Build history of the part. All positions in model axes, mm. A direction names the side the tool comes from. Give positions to 0.01 mm unless a question says otherwise; leave off trailing zeros. Order: outer loops, then holes, each group sorted by start corner. A loop starts at its lowest first (then second) coordinate and runs counter-clockwise, first axis right, second up. Notation, with made-up numbers: M -19.75,48.5 L 23.25,48.5 A18 ccw 23.25,72.5 Z; hole C -33,-37.5 d6. An arc over 180 degrees is marked long. Use CSV: the item, a comma, the result in double quotes. Start each with the question number.
Item 1: Band-saw the part on A-A on z = 0. Write the cut outline in (x, y).
Item 2: Band-saw the part on D-D on x = -32.5. Write the cut outline in (y, z), plus the area to 3 significant figures.
Item 3: Which spindle directions (+Z, -Z, +X, -X, +Y, -Y) get a long thin tool onto all of the face, cutting with end or side? Do faces 1 (the flat face through (19, 50.737, -19)), 2 (the cylindrical face through (0.1, 52.2, -28.5)), 3 (the conical face through (-12.376, 30.541, 3.897)). Say none if no direction does.
Item 4: Two-plate mould, pull along X, no slides. Class faces 4 (the cylindrical face through (-15.41, 56.78, -15.7)), 5 (the cylindrical face through (15.1, 56.8, 16)), 6 (the cylindrical face through (-28.5, 52.2, -0.1)): pulls with the +X half, pulls with the -X half, needs draft (parallel to the pull), parting line crosses it, or undercut.
Item 5: Wall check: line 1 along Z through (x, y) = (0, 54.25); line 2 along Z through (x, y) = (0, 12); line 3 along Y through (x, z) = (-28, -3). Give the ranges that are in metal, low to high.
Item 6: Band-saw the part on C-C on y = 9.5. Write the cut outline in (x, z), plus the area to 3 significant figures.
Item 7: Band-saw the part on B-B on x = 0. Write the cut outline in (y, z), plus the area to 3 significant figures.
Item 8: Pin check, flat tips, straight feed: P1, Ø1.4, axis at y = 52.5, z = -24, coming from the +X side; P2, Ø1.5, axis at y = 13, z = 9.5, coming from the -X side; P3, Ø12, axis at y = 14, z = 7, coming from the -X side. Stop position of each tip, or through.
from build123d import *

# Parameters (mm, degrees)
CUT_EXTRUDE1_START = -10
CUT_EXTRUDE1_DEPTH = 16
CIRPATTERN1_COUNT  = 2
CIRPATTERN1_ANGLE  = 90


with BuildPart() as part:
    # Sketch1 → Revolve1 (revolve)
    with BuildSketch(Plane.XY):
        with BuildLine():
            Line((-6.832916656, 22.5), (-6.832916656, 0))
            Line((-6.832916656, 0), (-8.332916656, 0))
            ThreePointArc((-8.332916656, 0), (-14, 11.25), (-8.332916656, 22.5))
            Line((-8.332916656, 22.5), (-24.635499254, 50.736901354))
            Line((-24.635499254, 50.736901354), (-45, 50.736901354))
            Line((-45, 50.736901354), (-45, 53.736901354))
            Line((-45, 53.736901354), (-22, 53.736901354))
            Line((-22, 53.736901354), (-22, 59.736901354))
            Line((-22, 59.736901354), (-20, 59.736901354))
            Line((-20, 59.736901354), (-20, 50.736901354))
            Line((-20, 50.736901354), (-6.832916656, 22.5))
        make_face()
    revolve(axis=Axis((0, -17.773369394, 0), (0, 1, 0)))

    # Sketch2 → Cut-Extrude1 (cut)
    with BuildSketch(Plane(origin=(0, 53.736901354, 0), x_dir=(1, 0, 0), z_dir=(0, 1, 0)).offset(CUT_EXTRUDE1_START)):
        with BuildLine():
            Line((-23.75, 3), (-25.5, 3))
            ThreePointArc((-25.5, 3), (-28.5, 0), (-25.5, -3))
            Line((-25.5, -3), (-23.75, -3))
            ThreePointArc((-23.75, -3), (-22.756426336, -2.830690971), (-21.875, -2.341874249))
            ThreePointArc((-21.875, -2.341874249), (-22, 0), (-21.875, 2.341874249))
            ThreePointArc((-21.875, 2.341874249), (-22.756426336, 2.830690971), (-23.75, 3))
        make_face()
        with BuildLine():
            ThreePointArc((-21.875, -2.341874249), (-20.75, 0), (-21.875, 2.341874249))
            ThreePointArc((-21.875, 2.341874249), (-22, 0), (-21.875, -2.341874249))
        make_face()
    cut_extrude1 = extrude(amount=CUT_EXTRUDE1_DEPTH, mode=Mode.SUBTRACT)

    # CirPattern1: Cut-Extrude1 ×2 about axis
    cirpattern1_axis = Axis((0, 0, 0), (0, -1, 0))
    for i in range(1, CIRPATTERN1_COUNT):
        add(cut_extrude1.rotate(cirpattern1_axis, i * CIRPATTERN1_ANGLE / (CIRPATTERN1_COUNT - 1)), mode=Mode.SUBTRACT)


solid = part.part
Model answer:
1,outline,"M -45,50.74 L -28.5,50.74 L -28.5,53.74 L -45,53.74 Z; M -20.75,44.01 L -8.33,22.5 A14 ccw -8.33,0 L -6.83,0 L -6.83,22.5 L -20,50.74 L -20,59.74 L -20.75,59.74 Z; M 6.83,0 L 8.33,0 A14 ccw 8.33,22.5 L 24.64,50.74 L 45,50.74 L 45,53.74 L 22,53.74 L 22,59.74 L 20,59.74 L 20,50.74 L 6.83,22.5 Z"
2,outline,"M 50.74,-31.12 L 53.74,-31.12 L 53.74,31.12 L 50.74,31.12 Z"
2,area,"187 mm^2"
3,face 1,"-Y"
3,face 2,"+Y, -Y"
3,face 3,"none"
4,face 4,"pulls with the -X half"
4,face 5,"parting line crosses it"
4,face 6,"undercut"
5,line 1,"z = -20.75 to -20, 20 to 22"
5,line 2,"z = -13.98 to -6.83, 6.83 to 13.98"
5,line 3,"y = 50.74 to 53.74"
6,outline,"C 0,0 d27.78; hole C 0,0 d13.67"
6,area,"459 mm^2"
7,outline,"M 0,-8.33 A14 ccw 22.5,-8.33 L 44.01,-20.75 L 59.74,-20.75 L 59.74,-20 L 50.74,-20 L 22.5,-6.83 L 0,-6.83 Z; M 0,6.83 L 22.5,6.83 L 50.74,20 L 59.74,20 L 59.74,22 L 53.74,22 L 53.74,45 L 50.74,45 L 50.74,24.64 L 22.5,8.33 A14 ccw 0,8.33 Z; M 50.74,-45 L 53.74,-45 L 53.74,-28.5 L 50.74,-28.5 Z"
7,area,"549 mm^2"
8,P1,"stops at x = 38.5"
8,P2,"stops at x = -10.8"
8,P3,"stops at x = -13.92"
